Check sheet for the modelled part. Datum: model origin and axes. Units: mm. A direction names the side the tool comes from. Coordinates: 2 decimals unless noted, no trailing zeros. Loops run counter-clockwise (first coordinate to the right, second up) from the corner with the lowest first, then second, coordinate; pieces in that order, holes last. Notation, with made-up numbers: (79, 31.5) -> (100, 31.5) arc R24 ccw to (100, 45.5) -> close; hole circle Ø4 at (51, 33). An arc over 180 degrees is marked (long way). Use CSV: the item, a comma, the result in double quotes.
```python
from build123d import *

# Parameters (mm, degrees)
EXTRUDE_1_DEPTH          = 26
SKETCH_2_R               = 1
CUT_EXTRUDE_4_DEPTH      = 27
CUT_EXTRUDE_4_DEPTH_BACK = 30
SKETCH_3_W               = 20
SKETCH_3_H               = 22
CUT_EXTRUDE_5_DEPTH      = 30
CUT_EXTRUDE_5_DEPTH_BACK = 30


with BuildPart() as part:
    # 草圖1 → 填料-伸長1 (new body)
    with BuildSketch(Plane.XY):
        with BuildLine():
            Line((-28, 5), (28, 5))
            ThreePointArc((28, 5), (33, 0), (28, -5))
            Line((28, -5), (-28, -5))
            ThreePointArc((-28, -5), (-33, 0), (-28, 5))
        make_face()
    extrude(amount=EXTRUDE_1_DEPTH)

    # 草圖2 → 除料-伸長4 (cut, two sides)
    with BuildSketch(Plane.XY) as cut_extrude_4_sk:
        with Locations((-28, 0)):
            Circle(SKETCH_2_R)
        with Locations((28, 0)):
            Circle(SKETCH_2_R)
    extrude(amount=CUT_EXTRUDE_4_DEPTH, mode=Mode.SUBTRACT)
    extrude(cut_extrude_4_sk.sketch, amount=-CUT_EXTRUDE_4_DEPTH_BACK, mode=Mode.SUBTRACT)

    # 草圖3 → 除料-伸長5 (cut, two sides)
    with BuildSketch(Plane(origin=(0, 0, 0), x_dir=(1, 0, 0), z_dir=(0, 1, 0))) as cut_extrude_5_sk:
        with Locations((-23, -13)):
            Rectangle(SKETCH_3_W, SKETCH_3_H)
        with Locations((23, -13)):
            Rectangle(SKETCH_3_W, SKETCH_3_H)
    extrude(amount=CUT_EXTRUDE_5_DEPTH, mode=Mode.SUBTRACT)
    extrude(cut_extrude_5_sk.sketch, amount=-CUT_EXTRUDE_5_DEPTH_BACK, mode=Mode.SUBTRACT)


solid = part.part
```
1) Access from +Z, -Z, +X, -X, +Y, -Y to the whole of each face (thin tool, end or side, straight path). Record for faces 4 (the flat face through (23, 0, 2)), 5 (the flat face through (-13, 0, 13)), 6 (the flat face through (0, -5, 13)).
Answer below:
face 4,"+X, +Y, -Y"
face 5,"-X, +Y, -Y"
face 6,"+Z, -Z, +X, -X, -Y"
2) Thickness scan on line 1 along X through (y, z) = (0, 0.65); line 2 along Z through (x, y) = (16, -3.25); line 3 along Y through (x, z) = (28, 25.45). Record the ranges inside material, lowest first. Write a range as from..to.
Answer below:
line 1,"x = -33..-29, -27..27, 29..33"
line 2,"z = 0..2, 24..26"
line 3,"y = -5..-1, 1..5"
3) Cross-section at C-C on y = 2.75. Record the boundary of the cut face in (x, z).
Answer below:
outline,"(-32.18, 0) -> (32.18, 0) -> (32.18, 2) -> (13, 2) -> (13, 24) -> (32.18, 24) -> (32.18, 26) -> (-32.18, 26) -> (-32.18, 24) -> (-13, 24) -> (-13, 2) -> (-32.18, 2) -> close"
4) Go/stop test with flat-tipped pins: pin 1 Ø1.8 at (x, y) = (28, 0) entering from -Z; pin 2 Ø2 at (y, z) = (1.5, 20.5) entering from +X; pin 3 Ø1 at (y, z) = (3, 18) entering from -X. Record where each tip stops, or that it passes through.
Answer below:
pin 1,"passes through"
pin 2,"stops at x = 13"
pin 3,"stops at x = -13"
5) Cross-section at A-A on y = 0. Record the boundary of the cut face in (x, z).
Answer below:
outline,"(-33, 0) -> (-29, 0) -> (-29, 2) -> (-33, 2) -> close; (-33, 24) -> (-29, 24) -> (-29, 26) -> (-33, 26) -> close; (-27, 0) -> (27, 0) -> (27, 2) -> (13, 2) -> (13, 24) -> (27, 24) -> (27, 26) -> (-27, 26) -> (-27, 24) -> (-13, 24) -> (-13, 2) -> (-27, 2) -> close; (29, 0) -> (33, 0) -> (33, 2) -> (29, 2) -> close; (29, 24) -> (33, 24) -> (33, 26) -> (29, 26) -> close"
6) Draft check along Z on faces 1 (the flat face through (23, 0, 24)), 2 (the cylindrical face through (-29, 0, 25)), 3 (the flat face through (0, 0, 0)). Enter one of: released by +Z, released by -Z, zero draft, split by the parting line, or undercut.
Answer below:
face 1,"undercut"
face 2,"zero draft"
face 3,"released by -Z"
7) Cross-section at B-B on x = -24. Record the boundary of the cut face in (y, z), and give its area (3 significant figures).
Answer below:
outline,"(-5, 0) -> (5, 0) -> (5, 2) -> (-5, 2) -> close; (-5, 24) -> (5, 24) -> (5, 26) -> (-5, 26) -> close"
area,"40.0 mm²"
8) Cross-section at D-D on z = 9.75. Record the boundary of the cut face in (x, y).
Answer below:
outline,"(-13, -5) -> (13, -5) -> (13, 5) -> (-13, 5) -> close"
